Read the model definition and answer for the solid it produces. Units are mm, in the model's axes. A direction names the side the tool comes from. Give positions to 0.01 mm unless a question says otherwise; leave off trailing zeros. Loops run counter-clockwise (first coordinate to the right, second up) from the corner with the lowest first, then second, coordinate; pieces in that order, holes last. Notation, with made-up numbers: (50.5, 69) -> (76.5, 69) arc R23 cw to (76.5, 92) -> close; hole circle Ø11 at (9, 87). An arc over 180 degrees is marked (long way). One line per item, written item: value. Start each with the question number.
from build123d import *

# Parameters (mm, degrees)
F0_R          = 0.5
F1_DEPTH      = 10
F0_R_2        = 1
F2_DEPTH      = 0.25
F3_R          = 0.15
F5_DEPTH      = 25
F5_DEPTH_BACK = 25
F7_DEPTH      = 25
F7_DEPTH_BACK = 25


with BuildPart() as f1:
    # F0 (on Top) → F1 (new body)
    with BuildSketch(Plane.XY):
        Circle(F0_R)
    extrude(amount=F1_DEPTH)

    # F0 (on Top) → F2 (join)
    with BuildSketch(Plane.XY):
        Circle(F0_R_2)
        Circle(F0_R, mode=Mode.SUBTRACT)
        Circle(F0_R)
    extrude(amount=-F2_DEPTH)

    # F3
    f3_edges = [f1.edges().sort_by_distance(p)[0] for p in [
        (-1, 0, -0.25),
    ]]
    fillet(f3_edges, radius=F3_R)

    # F4 (on Right) → F5 (cut, two sides)
    with BuildSketch(Plane.YZ) as f5_sk:
        Polygon((-0.5701061455, 9.0645924211), (0, 10.0047653541), (0.5819916259, 9.0299136937), (0.5819916259, 10.0856823847), (-0.6548758829, 10.0856823847), align=None)
    extrude(amount=F5_DEPTH, mode=Mode.SUBTRACT)
    extrude(f5_sk.sketch, amount=-F5_DEPTH_BACK, mode=Mode.SUBTRACT)

    # F6 (on Front) → F7 (cut, two sides)
    with BuildSketch(Plane.XZ) as f7_sk:
        Polygon((-0.5932200584, 9.1788349673), (0, 9.9986912683), (0.5793294404, 9.1912103817), (0.6381116109, 10.2987894788), (-0.5932200584, 10.2987894788), align=None)
    extrude(amount=F7_DEPTH, mode=Mode.SUBTRACT)
    extrude(f7_sk.sketch, amount=-F7_DEPTH_BACK, mode=Mode.SUBTRACT)


solid = f1.part
Item 1: Section A-A, the plane z = 4 is taken. Determine the outline of the cut face in (x, y), plus the area to 3 significant figures.
Item 2: For faces 1 (the flat face through (0, 0, -0.25)), 2 (the cylindrical face through (-0.108, -0.488, 4.669)), determine the directions among +Z, -Z, +X, -X, +Y, -Y from which every point of the face is accessible in a straight line to the end or side of a thin tool.
Item 3: Consider L1, parallel to Z at x = -0.7, y = 0.5; L2, parallel to Y at x = 0.2, z = 8.75; L3, parallel to X at y = 0.15, z = 9.25. Determine where each line is inside the solid, lowest interval first. Write a range as [from, to].
Item 4: A flat-ended cylindrical pin translates along its axis: pin 1 (0.6 mm diameter, centred on x = -0.5, y = -0.5, fed in from +Z). Find the tip coordinate at first contact, or state that the pin passes through.
Computed values:
1. outline: circle Ø1 at (0, 0)
1. area: 0.785 mm²
2. face 1: -Z, +X, -X, +Y, -Y
2. face 2: +Z
3. L1: [-0.25, 0]
3. L2: [-0.46, 0.46]
3. L3: [-0.48, 0.48]
4. pin 1: z = 9.57
